For this review, take the finished solid that the model builds, in its own axes (mm). Face numbers are marked on the shaded views. A direction names the side the tool comes from. Round coordinates to 2 decimals unless told otherwise and drop trailing zeros. Order: outer loops, then holes, each group sorted by start corner. A loop starts at its lowest first (then second) coordinate and runs counter-clockwise, first axis right, second up. Notation, with made-up numbers: (1, 34) -> (41, 34) arc R23 cw to (41, 52) -> close; hole circle Ø9 at (57, 76). An arc over 180 degrees is marked (long way). Use a Markdown table: item, result. Add a question column.
1) Machinability: for the marked faces 4, 5 and 6, which of the approach directions +Z, -Z, +X, -X, +Y, -Y give a long, thin tool a straight path to every point of the face, cutting with its end or side? Answer none if there is none.
2) Consider section A-A (x = 12.7). State the section outline as (y, z) points, plus the area to 3 significant figures.
3) Consider section D-D (y = -12.7). Give the number of separate pieces and of enclosed holes in the cut face, plus the area to 3 significant figures.
4) Consider section B-B (x = 121). State the section outline as (y, z) points.
5) Wall thickness on line 1 along X through (y, z) = (-60, 10.5); line 2 along Y through (x, z) = (12.7, 9); line 3 along X through (y, z) = (-68, 3.5): over which ranges is each line inside the solid? List them lowest first. Write a range as [from, to].
6) Draft analysis for pull direction Y (two halves, no side actions). For the marked faces 1, 2 and 3, state which applies: pulls with the +Y half, pulls with the -Y half, needs draft (parallel to the pull), parting line crosses it, or undercut.
7) Clearance check with flat-ended pins moving along their axes: P1, Ø4, axis at x = 12.7, y = -42.74, coming from the -Z side; P2, Ø6, axis at x = 92.5, y = -14.5, coming from the -Z side; P3, Ø4, axis at y = -63.5, z = 9, coming from the -X side; P4, Ø3, axis at x = 71, z = 6, coming from the +Y side. State where each tip first meets the part, or that it passes through.
8) Consider section C-C (y = -38). State the section outline as (x, z) points, plus the area to 3 significant figures.
```python
from build123d import *

# Parameters (mm, degrees)
BOSS_EXTRUDE1_DEPTH = 12.7
SKETCH2_R           = 2.54
SKETCH2_W           = 19.05
SKETCH2_H           = 55.44118298
CUT_EXTRUDE2_DEPTH  = 149.871187129
SKETCH3_W           = 100
SKETCH3_H           = 12.958545622
CUT_EXTRUDE3_DEPTH  = 149.871187129
SKETCH5_W           = 100
SKETCH5_H           = 9.525
BOSS_EXTRUDE3_DEPTH = 12.7
SKETCH4_R           = 2.24536
CUT_EXTRUDE4_DEPTH  = 154.464616373
SKETCH6_R           = 4.091253385
SKETCH6_R_2         = 6.05236999
SKETCH6_W           = 12.7
SKETCH6_H           = 25.4
BOSS_EXTRUDE4_DEPTH = 12.7
SKETCH7_R           = 2.54
CUT_EXTRUDE5_DEPTH  = 154.464616373
CUT_EXTRUDE6_DEPTH  = 154.464616373
SKETCH9_R           = 2.54
CUT_EXTRUDE7_DEPTH  = 9.525


with BuildPart() as part:
    # Sketch1 → Boss-Extrude1 (new body)
    with BuildSketch(Plane.XY):
        Polygon((31.75, -68.141601517), (31.75, -55.44118298), (0, -55.44118298), (0, -30.04118298), (19.05, -30.04118298), (31.75, -30.04118298), (31.75, -25.4), (19.05, -25.4), (0, -25.4), (0, 0), (19.05, 0), (31.75, 0), (131.75, -15.838444032), (131.75, -68.141601517), align=None)
    extrude(amount=BOSS_EXTRUDE1_DEPTH)

    # Sketch2 → Cut-Extrude2 (cut, through all)
    with BuildSketch(Plane.XY.offset(12.7)):
        with Locations((25.4, -12.7)):
            Circle(SKETCH2_R)
        with Locations(Location((25.4, -42.74118298, 0), (0, 0, 180))):
            Circle(SKETCH2_R)
        with Locations((9.525, -27.72059149)):
            Rectangle(SKETCH2_W, SKETCH2_H)
    extrude(amount=-CUT_EXTRUDE2_DEPTH, mode=Mode.SUBTRACT)

    # Sketch3 → Cut-Extrude3 (cut, through all)
    with BuildSketch(Plane.XY.offset(12.7)):
        with Locations((81.75, -74.620455791)):
            Rectangle(SKETCH3_W, SKETCH3_H)
    extrude(amount=-CUT_EXTRUDE3_DEPTH, mode=Mode.SUBTRACT)

    # Sketch5 → Boss-Extrude3 (add)
    with BuildSketch(Plane.XY.offset(12.7)):
        with Locations((81.75, -72.90368298)):
            Rectangle(SKETCH5_W, SKETCH5_H)
    extrude(amount=-BOSS_EXTRUDE3_DEPTH)

    # Sketch4 → Cut-Extrude4 (cut, through all)
    with BuildSketch(Plane.XY.offset(12.7)):
        with BuildLine():
            ThreePointArc((53.575418537, -55.44118298), (50.399790718, -55.440973698), (50.4, -58.616601517))
            Line((50.4, -58.616601517), (50.4, -55.44118298))
            Line((50.4, -55.44118298), (53.575418537, -55.44118298))
        make_face()
        with BuildLine():
            Line((50.4, -55.44118298), (50.4, -58.616601517))
            ThreePointArc((50.4, -58.616601517), (52.846898781, -59.103068495), (54.23286, -57.02868298))
            ThreePointArc((54.23286, -57.02868298), (54.06199877, -56.169557621), (53.575418537, -55.44118298))
            Line((53.575418537, -55.44118298), (50.4, -55.44118298))
        make_face()
        with Locations((61.5125, -57.02868298)):
            Circle(SKETCH4_R)
        with Locations((51.9875, -57.02868298)):
            Circle(SKETCH4_R)
        with Locations((51.9875, -66.55368298)):
            Circle(SKETCH4_R)
        with Locations((61.5125, -66.55368298)):
            Circle(SKETCH4_R)
        Polygon((63.1, -68.14118298), (63.1, -55.44118298), (56.75, -55.44118298), (50.4, -55.44118298), (50.4, -68.14118298), (56.75, -68.14118298), align=None)
        with BuildLine():
            ThreePointArc((59.924581463, -55.44118298), (59.924790718, -58.616392262), (63.1, -58.616601517))
            Line((63.1, -58.616601517), (63.1, -55.44118298))
            Line((63.1, -55.44118298), (59.924581463, -55.44118298))
        make_face()
        with BuildLine():
            Line((63.1, -55.44118298), (63.1, -58.616601517))
            ThreePointArc((63.1, -58.616601517), (63.586885515, -57.888081761), (63.75786, -57.02868298))
            ThreePointArc((63.75786, -57.02868298), (62.371625359, -54.95418421), (59.924581463, -55.44118298))
            Line((59.924581463, -55.44118298), (63.1, -55.44118298))
        make_face()
        with BuildLine():
            ThreePointArc((63.1, -64.965764443), (59.924790718, -64.965973698), (59.924581463, -68.14118298))
            Line((59.924581463, -68.14118298), (63.1, -68.14118298))
            Line((63.1, -68.14118298), (63.1, -64.965764443))
        make_face()
        with BuildLine():
            Line((63.1, -68.14118298), (59.924581463, -68.14118298))
            ThreePointArc((59.924581463, -68.14118298), (62.371625359, -68.62818175), (63.75786, -66.55368298))
            ThreePointArc((63.75786, -66.55368298), (63.586885515, -65.694284199), (63.1, -64.965764443))
            Line((63.1, -64.965764443), (63.1, -68.14118298))
        make_face()
        with BuildLine():
            ThreePointArc((50.4, -64.965764443), (50.399790718, -68.141392262), (53.575418537, -68.14118298))
            Line((53.575418537, -68.14118298), (50.4, -68.14118298))
            Line((50.4, -68.14118298), (50.4, -64.965764443))
        make_face()
        with BuildLine():
            Line((50.4, -68.14118298), (53.575418537, -68.14118298))
            ThreePointArc((53.575418537, -68.14118298), (54.06199877, -67.412808338), (54.23286, -66.55368298))
            ThreePointArc((54.23286, -66.55368298), (52.846898781, -64.479297465), (50.4, -64.965764443))
            Line((50.4, -64.965764443), (50.4, -68.14118298))
        make_face()
        with Locations((111.5125, -57.02868298)):
            Circle(SKETCH4_R)
        with Locations((101.9875, -57.02868298)):
            Circle(SKETCH4_R)
        with Locations((101.9875, -66.55368298)):
            Circle(SKETCH4_R)
        with Locations((111.5125, -66.55368298)):
            Circle(SKETCH4_R)
        Polygon((113.1, -68.14118298), (113.1, -55.44118298), (106.75, -55.44118298), (100.4, -55.44118298), (100.4, -68.14118298), (106.75, -68.14118298), align=None)
    extrude(amount=-CUT_EXTRUDE4_DEPTH, mode=Mode.SUBTRACT)

    # Sketch6 → Boss-Extrude4 (add)
    with BuildSketch(Plane.XY.offset(12.7)):
        with Locations((25.4, -12.7)):
            Circle(SKETCH6_R)
        with Locations((25.4, -42.74118298)):
            Circle(SKETCH6_R_2)
        with Locations((12.7, -12.7)):
            Rectangle(SKETCH6_W, SKETCH6_H)
        with Locations((12.7, -42.74118298)):
            Rectangle(SKETCH6_W, SKETCH6_H)
    extrude(amount=-BOSS_EXTRUDE4_DEPTH)

    # Sketch7 → Cut-Extrude5 (cut, through all)
    with BuildSketch(Plane.XY.offset(12.7)):
        with Locations((12.7, -12.7)):
            Circle(SKETCH7_R)
        with Locations(Location((12.7, -42.74118298, 0), (0, 0, 180))):
            Circle(SKETCH7_R)
    extrude(amount=-CUT_EXTRUDE5_DEPTH, mode=Mode.SUBTRACT)

    # Sketch8 → Cut-Extrude6 (cut, through all)
    with BuildSketch(Plane.XY.offset(12.7)):
        Polygon((131.75, -46.752313506), (131.75, -27.702313506), (119.05, -27.702313506), (119.05, -46.752313506), (119.05, -53.102313506), (131.75, -53.102313506), align=None)
    extrude(amount=-CUT_EXTRUDE6_DEPTH, mode=Mode.SUBTRACT)

    # Sketch9 → Cut-Extrude7 (cut)
    with BuildSketch(Plane(origin=(0.776977804, 4.905644786, 0), x_dir=(0.9876883405951382, -0.15643446504022795, 0), z_dir=(0.15643446504022795, 0.9876883405951383, 0))):
        with Locations(Location((81.982361103, -6.35, 0), (0, 0, 180))):
            Circle(SKETCH9_R)
    extrude(amount=-CUT_EXTRUDE7_DEPTH, mode=Mode.SUBTRACT)


solid = part.part
```
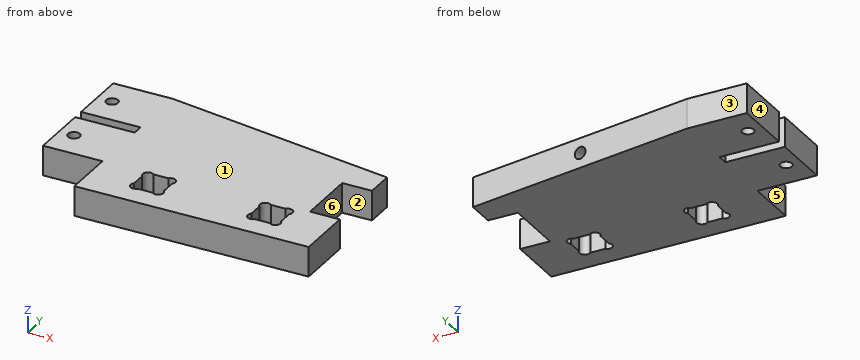
Results list:
| question | item | result |
|---|---|---|
| 1 | face 4 | +Z, -Z, -X, +Y, -Y |
| 1 | face 5 | +Z, -Z, -X, -Y |
| 1 | face 6 | +Z, -Z, +X |
| 2 | outline | (-55.44, 0) -> (-45.28, 0) -> (-45.28, 12.7) -> (-55.44, 12.7) -> close; (-40.2, 0) -> (-30.04, 0) -> (-30.04, 12.7) -> (-40.2, 12.7) -> close; (-25.4, 0) -> (-15.24, 0) -> (-15.24, 12.7) -> (-25.4, 12.7) -> close; (-10.16, 0) -> (0, 0) -> (0, 12.7) -> (-10.16, 12.7) -> close |
| 2 | area | 516 mm2 |
| 3 | separate pieces | 2 |
| 3 | enclosed holes | 1 |
| 3 | area | 1,260 mm2 |
| 4 | outline | (-77.67, 0) -> (-53.1, 0) -> (-53.1, 12.7) -> (-77.67, 12.7) -> close; (-27.7, 0) -> (-14.14, 0) -> (-14.14, 12.7) -> (-27.7, 12.7) -> close |
| 5 | line 1 | [31.75, 50.4], [63.1, 100.4], [113.1, 131.75] |
| 5 | line 2 | [-55.44, -45.28], [-40.2, -30.04], [-25.4, -15.24], [-10.16, 0] |
| 5 | line 3 | [31.75, 50.27], [63.23, 100.27], [113.23, 131.75] |
| 6 | face 1 | needs draft |
| 6 | face 2 | undercut |
| 6 | face 3 | pulls with the +Y half |
| 7 | P1 | through |
| 7 | P2 | z = 0 |
| 7 | P3 | x = 31.75 |
| 7 | P4 | y = -5.98 |
| 8 | outline | (6.35, 0) -> (119.05, 0) -> (119.05, 12.7) -> (6.35, 12.7) -> close |
| 8 | area | 1,430 mm2 |
